Geometry check sheet. Reference: the model listing, model coordinates, mm. A direction names the side the tool comes from. Give positions to 0.01 mm unless a question says otherwise; leave off trailing zeros. Write each loop counter-clockwise with the first axis right and the second up, starting at its lowest first coordinate (ties: lowest second). Pieces come first, ordered by that corner, then holes.
(1) Cross-section at A-A (x = 0). Record the boundary of the cut face in (y, z) (1 decimal).
(2) Thickness scan on line 1 along Z through (x, y) = (0, 11.75) (1 decimal); line 2 along Y through (x, z) = (1, -6); line 3 along Z through (x, y) = (0.25, 2.5) (3 decimals). Record the ranges inside material, lowest first.
(3) Mould release check, pull along Y, two halves, no side actions. Record for faces 4 (the flat face through (0, 0, -4)), 5 (the flat face through (0, 14, -7.144)), 6 (the flat face through (-2.668, 14.566, -8.238)): +Y half, -Y half, draft (parallel to the pull), parting line (faces both ways), or undercut.
(4) Cross-section at B-B (y = 13.75). Count the separate pieces of the cut face and the enclosed holes in it, and give its area (3 significant figures).
(5) Depth check by flat-ended pin: P1, Ø1.7, axis at x = 1, y = 2.5, coming from the +Z side; P2, Ø0.5, axis at x = -1, y = 14.5, coming from the +Z side; P3, Ø5, axis at y = 5, z = -4.5, coming from the +X side (3 decimals); P4, Ø1.5, axis at y = 14.5, z = 1.5, coming from the +X side. Enter the tip coordinate at first touch or a pass-through.
(6) Cross-section at C-C (z = -3.5). Record the boundary of the cut face in (x, y) (1 decimal).
(7) Tool access check on faces 1 (the flat face through (0, 3.175, -8)), 2 (the flat face through (0, 2, -7.144)), 3 (the flat face through (-2.557, 15.985, -8.033)). Record the directions out of +Z, -Z, +X, -X, +Y, -Y that give a thin tool (end or side, any length) a straight path to the whole face; none if there is none.
```python
from build123d import *

# Parameters (mm, degrees)
SKETCH1_R           = 1.5875
BOSS_EXTRUDE1_DEPTH = 16.66875
CUT_EXTRUDE1_DEPTH  = 7.35
CHAMFER1_SIZE       = 1


with BuildPart() as part:
    # Sketch1 → Boss-Extrude1 (new body)
    with BuildSketch(Plane(origin=(0, 0, 0), x_dir=(1, 0, 0), z_dir=(0, 1, 0))):
        with BuildLine():
            Line((-3.175, 0), (-3.175, 8.73125))
            Line((-3.175, 8.73125), (3.175, 8.73125))
            Line((3.175, 8.73125), (3.175, 0))
            ThreePointArc((3.175, 0), (0, -3.175), (-3.175, 0))
        make_face()
        Circle(SKETCH1_R, mode=Mode.SUBTRACT)
    extrude(amount=BOSS_EXTRUDE1_DEPTH)

    # Sketch3 → Cut-Extrude1 (cut, through all)
    with BuildSketch(Plane(origin=(3.175, 0, 0), x_dir=(0, 0, -1), z_dir=(1, 0, 0))):
        Polygon((8.73125, 13.49375), (7.14375, 13.49375), (7.14375, 15.08125), (3.175, 15.08125), (3.175, 1.5875), (7.14375, 1.5875), (7.14375, 3.175), (8.73125, 3.175), align=None)
    extrude(amount=-CUT_EXTRUDE1_DEPTH, mode=Mode.SUBTRACT)

    # Chamfer1
    chamfer1_edges = [part.edges().sort_by_distance(p)[0] for p in [
        (0, 16.66875, -8.73125),
        (-3.175, 16.66875, -4.365625),
        (-3.175, 1.5875, -8.73125),
        (3.175, 1.5875, -8.73125),
        (0, 16.66875, 3.175),
        (-3.175, 0, -4.365625),
        (0, 0, -8.73125),
        (3.175, 0, -4.365625),
        (0, 0, 3.175),
        (3.175, 16.66875, -4.365625),
        (-3.175, 15.08125, -8.73125),
        (3.175, 15.08125, -8.73125),
    ]]
    chamfer(chamfer1_edges, length=CHAMFER1_SIZE)


solid = part.part
```
Reply:
1. outline: (0, -7.7) - (1, -8.7) - (3.2, -8.7) - (3.2, -7.1) - (1.6, -7.1) - (1.6, -3.2) - (15.1, -3.2) - (15.1, -7.1) - (13.5, -7.1) - (13.5, -8.7) - (15.7, -8.7) - (16.7, -7.7) - (16.7, -1.6) - (0, -1.6) - close; (0, 1.6) - (16.7, 1.6) - (16.7, 2.2) - (15.7, 3.2) - (1, 3.2) - (0, 2.2) - close
2. line 1: z = -3.2 to -1.6, 1.6 to 3.2
2. line 2: y = 0 to 1.59, 15.08 to 16.67
2. line 3: z = -8.731 to -7.144, -3.175 to -1.568, 1.568 to 3.165
3. face 4: -Y half
3. face 5: undercut
3. face 6: draft
4. separate pieces: 2
4. enclosed holes: 1
4. area: 37.2 mm2
5. P1: stops at z = 3.17
5. P2: stops at z = 3.09
5. P3: stops at x = 3.175
5. P4: stops at x = 3.09
6. outline: (-3.2, 1) - (-2.2, 0) - (2.2, 0) - (3.2, 1) - (3.2, 1.6) - (-3.2, 1.6) - close; (-3.2, 15.1) - (3.2, 15.1) - (3.2, 15.7) - (2.2, 16.7) - (-2.2, 16.7) - (-3.2, 15.7) - close
7. face 1: -Z, +X, -X
7. face 2: +X, -X
7. face 3: -Z, -X, +Y
